Source: CAD feature listing. Evaluate the final solid. Frame: model axes, mm. Face numbers are marked on the shaded views. A direction names the side the tool comes from. Round coordinates to 2 decimals unless told otherwise and drop trailing zeros. Loops run counter-clockwise (first coordinate to the right, second up) from the corner with the lowest first, then second, coordinate; pieces in that order, holes last. Notation, with made-up numbers: (-39, 76.5) - (9, 76.5) arc R20 cw to (9, 85.5) - close; hole circle Ø9 at (84.25, 59). An arc over 180 degrees is marked (long way). Write item = value, one per line. Start each with the question number.
from build123d import *

# Parameters (mm, degrees)
SKETCH_1_W          = 86.3
SKETCH_1_H          = 33.5
EXTRUDE_1_DEPTH     = 13
EXTRUDE_2_DEPTH     = 13
SKETCH_7_W          = 86.3
SKETCH_7_H          = 7
CUT_EXTRUDE_3_DEPTH = 3
SKETCH_8_W          = 86.3
SKETCH_8_H          = 7
CUT_EXTRUDE_4_DEPTH = 30
SKETCH_9_R          = 0.975
CUT_EXTRUDE_5_DEPTH = 58.992865941
SKETCH_10_W         = 4
SKETCH_10_H         = 4
CUT_EXTRUDE_6_DEPTH = 50.203505973


with BuildPart() as part:
    # ｽｹｯﾁ1 → ﾎﾞｽ - 押し出し1 (new body)
    with BuildSketch(Plane.XY):
        Rectangle(SKETCH_1_W, SKETCH_1_H)
    extrude(amount=EXTRUDE_1_DEPTH)

    # ｽｹｯﾁ3 → ﾎﾞｽ - 押し出し2 (add)
    with BuildSketch(Plane(origin=(0, 0, 0), x_dir=(-1, 0, 0), z_dir=(0, 0, -1))):
        Polygon((-43.15, 16.75), (-43.15, 19.75), (-34.907567742, 16.75), align=None)
        Polygon((43.15, 16.75), (43.15, 19.75), (34.907567742, 16.75), align=None)
    extrude(amount=-EXTRUDE_2_DEPTH)

    # ｽｹｯﾁ7 → ｶｯﾄ - 押し出し3 (cut)
    with BuildSketch(Plane(origin=(0, 16.75, 0), x_dir=(1, 0, 0), z_dir=(0, 1, 0))):
        with Locations((0, -6.5)):
            Rectangle(SKETCH_7_W, SKETCH_7_H)
    extrude(amount=CUT_EXTRUDE_3_DEPTH, mode=Mode.SUBTRACT)

    # ｽｹｯﾁ8 → ｶｯﾄ - 押し出し4 (cut)
    with BuildSketch(Plane(origin=(0, 16.75, 0), x_dir=(1, 0, 0), z_dir=(0, 1, 0))):
        with Locations((0, -6.5)):
            Rectangle(SKETCH_8_W, SKETCH_8_H)
    extrude(amount=-CUT_EXTRUDE_4_DEPTH, mode=Mode.SUBTRACT)

    # ｽｹｯﾁ9 → ｶｯﾄ - 押し出し5 (cut, through all)
    with BuildSketch(Plane.XZ.offset(16.75)):
        with Locations((-38.15, 6.5)):
            Circle(SKETCH_9_R)
        with Locations((38.15, 6.5)):
            Circle(SKETCH_9_R)
    extrude(amount=-CUT_EXTRUDE_5_DEPTH, mode=Mode.SUBTRACT)

    # ｽｹｯﾁ10 → ｶｯﾄ - 押し出し6 (cut, through all)
    with BuildSketch(Plane.XY.offset(13)):
        with Locations((7.45, -14.75)):
            Rectangle(SKETCH_10_W, SKETCH_10_H)
        with Locations((19.15, -14.75)):
            Rectangle(SKETCH_10_W, SKETCH_10_H)
    extrude(amount=-CUT_EXTRUDE_6_DEPTH, mode=Mode.SUBTRACT)


solid = part.part
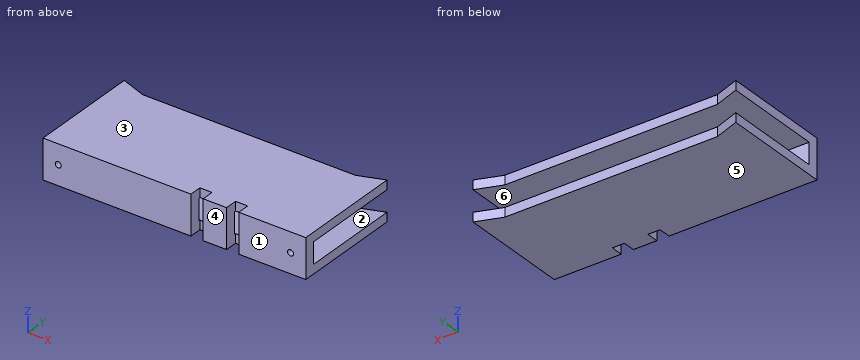
(1) Mould query, pull axis Z, two halves, no side actions, for the marked faces 3, 4, 5 and 6. Classes: +Z half, -Z half, draft (parallel to the pull), parting line (faces both ways), or undercut.
(2) Cut plane A-A (y = 15.5). Output: boundary loops of the cut face in (x, z), and give its area (3 significant figures).
(3) Pin query (flat end, axial travel): P1, Ø5.5, axis at x = 15, z = 5.5, coming from the +Y side; P2, Ø0.9, axis at x = 18.5, z = 12, coming from the -Y side. Return the tip coordinate at first contact, or that it passes through.
(4) Access query for the marked faces 1 and 2. Directions: +Z, -Z, +X, -X, +Y, -Y. A direction counts if a zero-diameter tool reaches every point of the face in a straight line with its end or side. Return the directions, or none.
(5) Cut plane D-D (z = 2). Output: boundary loops of the cut face in (x, y), and give its area (3 significant figures).
(6) Cut plane B-B (z = 6.5). Output: boundary loops of the cut face in (x, y) (3 decimals).
(7) Material intervals for line 1 along Z through (x, y) = (-12, -12.5); line 2 along Z through (x, y) = (-38.15, -15.3) (3 decimals); line 3 along X through (y, z) = (-14.5, 7.75), sorted ascending. Write a range as from..to.
(8) Cut plane C-C (x = 27). Output: boundary loops of the cut face in (y, z), and give its area (4 significant figures).
Solution:
q1.face_3 = +Z half
q1.face_4 = draft
q1.face_5 = -Z half
q1.face_6 = undercut
q2.outline = (-43.15, 0) - (43.15, 0) - (43.15, 3) - (-43.15, 3) - close; (-43.15, 10) - (43.15, 10) - (43.15, 13) - (-43.15, 13) - close
q2.area = 518 mm^2
q3.P1 = 16.75
q3.P2 = -12.75
q4.face_1 = +Z, -Z, +X, -X, -Y
q4.face_2 = +X, -X, +Y
q5.outline = (-43.15, -16.75) - (5.45, -16.75) - (5.45, -12.75) - (9.45, -12.75) - (9.45, -16.75) - (17.15, -16.75) - (17.15, -12.75) - (21.15, -12.75) - (21.15, -16.75) - (43.15, -16.75) - (43.15, 19.75) - (34.91, 16.75) - (-34.91, 16.75) - (-43.15, 19.75) - close
q5.area = 2,880 mm^2
q6.outline = (-43.15, -16.75) - (-39.125, -16.75) - (-39.125, -13.25) - (-43.15, -13.25) - close; (-37.175, -16.75) - (5.45, -16.75) - (5.45, -13.25) - (-37.175, -13.25) - close; (9.45, -16.75) - (17.15, -16.75) - (17.15, -13.25) - (9.45, -13.25) - close; (21.15, -16.75) - (37.175, -16.75) - (37.175, -13.25) - (21.15, -13.25) - close; (39.125, -16.75) - (43.15, -16.75) - (43.15, -13.25) - (39.125, -13.25) - close
q7.line_1 = 0..3, 10..13
q7.line_2 = 0..5.525, 7.475..13
q7.line_3 = -43.15..5.45, 9.45..17.15, 21.15..43.15
q8.outline = (-16.75, 0) - (16.75, 0) - (16.75, 3) - (-13.25, 3) - (-13.25, 10) - (16.75, 10) - (16.75, 13) - (-16.75, 13) - close
q8.area = 225.5 mm^2
